```python
from build123d import *

# Parameters (mm, degrees)
ESQUISSE1_W             = 83
ESQUISSE1_H             = 73
ESQUISSE1_R             = 7.5
BOSS_EXTRU_1_DEPTH      = 5
ESQUISSE2_R             = 1.5
ESQUISSE2_W             = 5
ESQUISSE2_H             = 6
ESQUISSE2_H_2           = 3.25
ESQUISSE2_H_3           = 5
ENL_V_MAT_EXTRU_1_DEPTH = 5
ESQUISSE3_W             = 20
ESQUISSE3_H             = 5
BOSS_EXTRU_2_DEPTH      = 5


with BuildPart() as part:
    # Esquisse1 → Boss.-Extru.1 (new body)
    with BuildSketch(Plane.XY):
        with Locations((41.5, 36.5)):
            Rectangle(ESQUISSE1_W, ESQUISSE1_H)
        with Locations((41.5, 31.275)):
            Circle(ESQUISSE1_R, mode=Mode.SUBTRACT)
    extrude(amount=BOSS_EXTRU_1_DEPTH)

    # Esquisse2 → Enlèv. mat.-Extru.1 (cut)
    with BuildSketch(Plane.XY.offset(5)):
        with Locations((41.5, 47.275)):
            Circle(ESQUISSE2_R)
        with Locations((25.5, 31.275)):
            Circle(ESQUISSE2_R)
        with Locations((57.5, 31.275)):
            Circle(ESQUISSE2_R)
        with Locations((41.5, 15.275)):
            Circle(ESQUISSE2_R)
        with Locations((80.5, 70)):
            Rectangle(ESQUISSE2_W, ESQUISSE2_H)
        with Locations((80.5, 54)):
            Rectangle(ESQUISSE2_W, ESQUISSE2_H)
        with Locations((80.5, 1.625)):
            Rectangle(ESQUISSE2_W, ESQUISSE2_H_2)
        with Locations((80.5, 9.875)):
            Rectangle(ESQUISSE2_W, ESQUISSE2_H_2)
        with Locations((2.5, 9.875)):
            Rectangle(ESQUISSE2_W, ESQUISSE2_H_2)
        with Locations((2.5, 1.625)):
            Rectangle(ESQUISSE2_W, ESQUISSE2_H_2)
        with Locations((2.5, 54)):
            Rectangle(ESQUISSE2_W, ESQUISSE2_H)
        with Locations((2.5, 70)):
            Rectangle(ESQUISSE2_W, ESQUISSE2_H)
        with Locations((20.016662646, 70.5)):
            Rectangle(ESQUISSE2_W, ESQUISSE2_H_3)
        with Locations((62.983337354, 70.5)):
            Rectangle(ESQUISSE2_W, ESQUISSE2_H_3)
    extrude(amount=-ENL_V_MAT_EXTRU_1_DEPTH, mode=Mode.SUBTRACT)

    # Esquisse3 → Boss.-Extru.2 (add)
    with BuildSketch(Plane.XY.offset(5)):
        with Locations((63, 75.5)):
            Rectangle(ESQUISSE3_W, ESQUISSE3_H)
        with Locations((20, 75.5)):
            Rectangle(ESQUISSE3_W, ESQUISSE3_H)
        with Locations((63, -2.5)):
            Rectangle(ESQUISSE3_W, ESQUISSE3_H)
        with Locations((20, -2.5)):
            Rectangle(ESQUISSE3_W, ESQUISSE3_H)
    extrude(amount=-BOSS_EXTRU_2_DEPTH)


solid = part.part
```
Geometry check sheet. Reference: the model listing, model coordinates, mm. A direction names the side the tool comes from. Coordinates: 2 decimals unless noted, no trailing zeros. Order: outer loops, then holes, each group sorted by start corner. A loop starts at its lowest first (then second) coordinate and runs counter-clockwise, first axis right, second up. Notation, with made-up numbers: M 61,29.25 L 81,29.25 A9 ccw 81,35.25 Z; hole C 49,-2.5 d6. An arc over 180 degrees is marked long. Answer as a JSON object with one key per item and string values.
Q1. Tool access check on faces 1 (the flat face through (75, 73, 2)), 2 (the flat face through (60.483, 70, 3)), 3 (the flat face through (5, 10, 3)), 4 (the flat face through (80, 57, 3)). Record the directions out of +Z, -Z, +X, -X, +Y, -Y that give a thin tool (end or side, any length) a straight path to the whole face; none if there is none.
Results are:
{"face 1": "+Z, -Z, +X, +Y", "face 2": "+Z, -Z", "face 3": "+Z, -Z, -X", "face 4": "+Z, -Z, +X"}
Q2. Depth check by flat-ended pin: pin 1 Ø1.5 at (x, z) = (81, 3) entering from +Y; pin 2 Ø1 at (x, z) = (74, 2.5) entering from +Y; pin 3 Ø1.5 at (y, z) = (-1.5, 1.5) entering from +X. Enter the tip coordinate at first touch or a pass-through.
Results are:
{"pin 1": "stops at y = 67", "pin 2": "stops at y = 73", "pin 3": "stops at x = 73"}
Q3. Release check for a two-part mould opening along X. For faces 5 (the flat face through (20, -5, 3)), 6 (the flat face through (53, -3, 3)), 7 (the flat face through (5, 2, 3)) record: released by +X, released by -X, zero draft, split by the parting line, or undercut.
Results are:
{"face 5": "zero draft", "face 6": "undercut", "face 7": "released by -X"}
Q4. Scan lines: line 1 (X direction, y = 70.5, z = 0.65); line 2 (Y direction, x = 41.5, z = 2.3) (3 decimals); line 3 (Y direction, x = 21.5, z = 2.05). Record each from-to range of solid material in increasing order.
Results are:
{"line 1": "x = 5 to 17.52, 22.52 to 60.48, 65.48 to 78", "line 2": "y = 0 to 13.775, 16.775 to 23.775, 38.775 to 45.775, 48.775 to 73", "line 3": "y = -5 to 68, 73 to 78"}
Q5. Cross-section at A-A on x = 41.5. Record the cut outline in (y, z) (3 decimals).
Results are:
{"outline": "M 0,0 L 13.775,0 L 13.775,5 L 0,5 Z; M 16.775,0 L 23.775,0 L 23.775,5 L 16.775,5 Z; M 38.775,0 L 45.775,0 L 45.775,5 L 38.775,5 Z; M 48.775,0 L 73,0 L 73,5 L 48.775,5 Z"}
Q6. Cross-section at B-B on x = 57.5. Record the cut outline in (y, z) (3 decimals).
Results are:
{"outline": "M -5,0 L 29.775,0 L 29.775,5 L -5,5 Z; M 32.775,0 L 78,0 L 78,5 L 32.775,5 Z"}
Q7. Cross-section at C-C on z = 2.85. Give the number of separate pieces and of enclosed holes in the cut face, and give its area (3 significant figures).
Results are:
{"separate pieces": "1", "enclosed holes": "7", "area": "6,020 mm²"}
